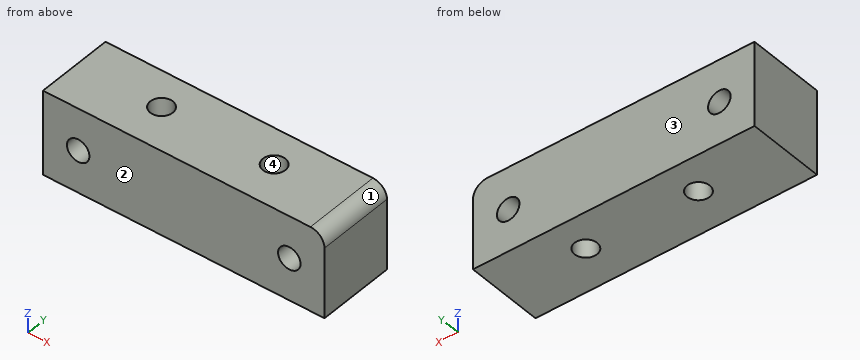
from build123d import *

# Parameters (mm, degrees)
SKETCH1_W             = 20
SKETCH1_H             = 6
BOSS_EXTRUDE1_DEPTH   = 5.5
M2X0_4_TAPPED_HOLE2_D = 1.6
FILLET1_R             = 1
M2X0_4_TAPPED_HOLE1_D = 1.6


with BuildPart() as part:
    # Sketch1 → Boss-Extrude1 (new body)
    with BuildSketch(Plane(origin=(0, 0, 0), x_dir=(1, 0, 0), z_dir=(0, 1, 0))):
        Rectangle(SKETCH1_W, SKETCH1_H)
    extrude(amount=-BOSS_EXTRUDE1_DEPTH)

    # M2x0.4 Tapped Hole2 (through all)
    with Locations(Plane(origin=(0, 0, 0), x_dir=(-1, 0, 0), z_dir=(0, 1, 0))):
        with Locations((7.5, 0), (-7.5, 0)):
            Hole(M2X0_4_TAPPED_HOLE2_D / 2)

    # Fillet1
    fillet1_edges = [part.edges().sort_by_distance(p)[0] for p in [
        (10, -2.75, 3),
    ]]
    fillet(fillet1_edges, radius=FILLET1_R)

    # M2x0.4 Tapped Hole1 (through all)
    with Locations(Plane.XY.offset(3)):
        with Locations((-4, -2.5), (4, -2.5)):
            Hole(M2X0_4_TAPPED_HOLE1_D / 2)


solid = part.part
Input: part model. Units: mm. Frame: model coordinates. Face numbers are marked on the shaded views. Coordinates: 2 decimals unless noted, no trailing zeros. Loops run counter-clockwise (first coordinate to the right, second up) from the corner with the lowest first, then second, coordinate; pieces in that order, holes last. Notation, with made-up numbers: (77, 51.25) -> (98, 51.25) arc R13 ccw to (98, 69.25) -> close; hole circle Ø10 at (63.25, 63.25). An arc over 180 degrees is marked (long way). Write each question's results on one line, items separated by ' | '. Start each with the question number.
Q1. Section C-C, the plane x = -7.5. Return the cut outline in (y, z), plus the area to 3 significant figures.
Q2. Section A-A, the plane y = -2.5. Return the cut outline in (x, z), plus the area to 3 significant figures.
Q3. Ray query, line 1 (X direction, y = -4.95, z = -0.05); line 2 (X direction, y = -2.2, z = -2.5); line 3 (Z direction, x = -7.5, y = -2.6). Return the intervals inside material, ascending. Write a range as from..to.
Q4. Section B-B, the plane z = -0.45. Return the cut outline in (x, y).
Q5. Section D-D, the plane y = -4.65. Return the cut outline in (x, z), plus the area to 3 significant figures.
Q6. Pull-direction query (Y, two-part tool) for the marked faces 1, 2, 3 and 4; classes: released by +Y, released by -Y, zero draft, split by the parting line, or undercut.
Found:
1) outline: (-5.5, -3) -> (0, -3) -> (0, -0.8) -> (-5.5, -0.8) -> close; (-5.5, 0.8) -> (0, 0.8) -> (0, 3) -> (-5.5, 3) -> close | area: 24.2 mm2
2) outline: (-10, -3) -> (-4.8, -3) -> (-4.8, 3) -> (-10, 3) -> close; (-3.2, -3) -> (3.2, -3) -> (3.2, 3) -> (-3.2, 3) -> close; (4.8, -3) -> (10, -3) -> (10, 2) arc R1 ccw to (9, 3) -> (4.8, 3) -> close; hole circle Ø1.6 at (-7.5, 0); hole circle Ø1.6 at (7.5, 0) | area: 96.6 mm2
3) line 1: -10..-8.3, -6.7..6.7, 8.3..10 | line 2: -10..-4.74, -3.26..3.26, 4.74..10 | line 3: -3..-0.8, 0.8..3
4) outline: (-10, -5.5) -> (-8.16, -5.5) -> (-8.16, 0) -> (-10, 0) -> close; (-6.84, -5.5) -> (6.84, -5.5) -> (6.84, 0) -> (-6.84, 0) -> close; (8.16, -5.5) -> (10, -5.5) -> (10, 0) -> (8.16, 0) -> close; hole circle Ø1.6 at (-4, -2.5); hole circle Ø1.6 at (4, -2.5)
5) outline: (-10, -3) -> (10, -3) -> (10, 2) arc R1 ccw to (9, 3) -> (-10, 3) -> close; hole circle Ø1.6 at (-7.5, 0); hole circle Ø1.6 at (7.5, 0) | area: 116 mm2
6) face 1: zero draft | face 2: released by -Y | face 3: released by +Y | face 4: undercut
